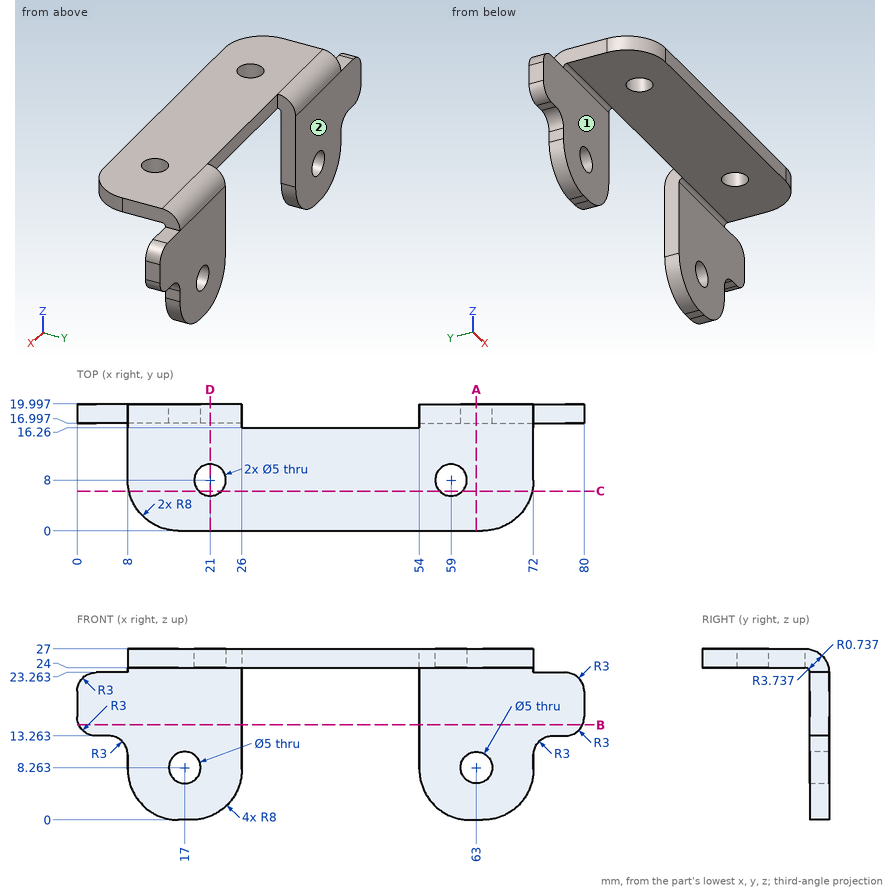
Study the drawing (mm; zero at the part's minimum x, y, z) and answer. A direction names the side the tool comes from. Coordinates: 2 decimals unless noted, no trailing zeros. Order: outer loops, then holes, each group sorted by start corner. A loop starts at its lowest first (then second) coordinate and runs counter-clockwise, first axis right, second up. Notation, with made-up numbers: M 87.5,73 L 132.5,73 A18 ccw 132.5,108 Z; hole C -10.75,43.25 d8. An arc over 180 degrees is marked long. Answer as a JSON object with one key per item and string values. Group by question number.
1. Section C-C on y = 6.25 is taken. Write down the section's boundary in (x, z) (1 decimal).
2. Section B-B on z = 15 is taken. Write down the section's boundary in (x, y), then the cut area to 3 significant figures.
3. Section D-D on x = 21 is taken. Write down the section's boundary in (y, z), then the cut area to 3 significant figures.
4. Flat-ended cylindrical pins translate along their axes: P1, Ø2, axis at x = 53.5, z = 8, coming from the -Y side; P2, Ø1.9, axis at y = 15, z = 26, coming from the -X side; P3, Ø1.5, axis at x = 41.5, z = 25.5, coming from the +Y side; P4, Ø6, axis at y = 12.5, z = 19, coming from the -X side. Find the tip coordinate at first contact, or state that the pin passes through.
5. Straight lines are drawn through the part: line 1 (X direction, y = 9.75, z = 25) (1 decimal); line 2 (Y direction, x = 57, z = 6); line 3 (X direction, y = 19, z = 17.25). For each, find the intervals that lie inside material, in ascending order.
6. Section A-A on x = 63 is taken. Write down the section's boundary in (y, z).
7. A tool of negligible diameter and unlimited length cuts with its end or side. For the marked faces 1 and 2, from which of +Z, -Z, +X, -X, +Y, -Y can it reach the whole face along a straight path? Write none if from no direction.
Values follow:
{
 "1": {"outline": "M 8.2,24 L 19.2,24 L 19.2,27 L 8.2,27 Z; M 22.8,24 L 57.2,24 L 57.2,27 L 22.8,27 Z; M 60.8,24 L 71.8,24 L 71.8,27 L 60.8,27 Z"},
 "2": {"outline": "M 0.28,17 L 26,17 L 26,20 L 0.28,20 Z; M 54,17 L 79.72,17 L 79.72,20 L 54,20 Z", "area": "154 mm2"},
 "3": {"outline": "M 0,24 L 5.5,24 L 5.5,27 L 0,27 Z; M 10.5,24 L 16.26,24 A0.74 cw 17,23.26 L 17,0.58 L 20,0.58 L 20,23.26 A3.74 ccw 16.26,27 L 10.5,27 Z", "area": "112 mm2"},
 "4": {"P1": "y = 17", "P2": "x = 8", "P3": "y = 16.26", "P4": "through"},
 "5": {"line 1": "8 to 19.2, 22.8 to 57.2, 60.8 to 72", "line 2": "17 to 20", "line 3": "0 to 26, 54 to 80"},
 "6": {"outline": "M 0,24 L 16.26,24 A0.74 cw 17,23.26 L 17,10.76 L 20,10.76 L 20,23.26 A3.74 ccw 16.26,27 L 0,27 Z; M 17,0 L 20,0 L 20,5.76 L 17,5.76 Z"},
 "7": {"face 1": "-Z, +X, -X, -Y", "face 2": "+Z, -Z, +X, -X, +Y"}
}
